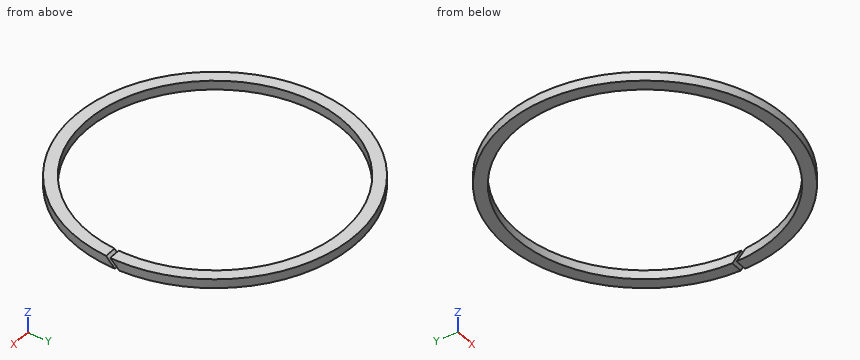
from build123d import *

# Parameters (mm, degrees)
SKETCH1_R               = 46.5
SKETCH1_R_2             = 42.5
BOSS_EXTRUDE1_DEPTH     = 3
CUT_EXTRUDE2_REACH      = 67.829
CUT_EXTRUDE2_END_RADIUS = 46.5


with BuildPart() as part:
    # Sketch1 → Boss-Extrude1 (new body)
    with BuildSketch(Plane.XY):
        Circle(SKETCH1_R)
        Circle(SKETCH1_R_2, mode=Mode.SUBTRACT)
    extrude(amount=BOSS_EXTRUDE1_DEPTH)

    # Cut-Extrude2: up to this cylinder (the profile starts inside it)
    cut_extrude2_end = Plane(origin=(0, 0, -0.237725), z_dir=(0, 0, -1)) * Cylinder(CUT_EXTRUDE2_END_RADIUS, 229.658, mode=Mode.PRIVATE)
    # Sketch2 → Cut-Extrude2 (cut, up to the surface)
    with BuildSketch(Plane(origin=(0, 0, 0), x_dir=(0, 0, -1), z_dir=(1, 0, 0)), mode=Mode.PRIVATE) as cut_extrude2_sk1:
        Polygon((-14.60888812, -13.901781339), (14.377231128, 15.08433791), (15.08433791, 14.377231128), (-13.901781339, -14.60888812), align=None)
    cut_extrude2_tool1 = extrude(cut_extrude2_sk1.sketch, amount=CUT_EXTRUDE2_REACH, mode=Mode.PRIVATE) & cut_extrude2_end
    add(cut_extrude2_tool1.solids().sort_by_distance((0, 0.237725, -0.237725))[0], mode=Mode.SUBTRACT)


solid = part.part
The listing builds one solid part. Answer for the finished solid, in the listing's coordinates (mm). Give positions to 0.01 mm unless a question says otherwise; leave off trailing zeros. Write each loop counter-clockwise with the first axis right and the second up, starting at its lowest first coordinate (ties: lowest second). Pieces come first, ordered by that corner, then holes.
Item 1: Find the intervals of material crossed by line 1 along Y through (x, z) = (0, 1.1); line 2 along Y through (x, z) = (6, 2.45), in increasing order.
Item 2: Section C-C, the plane z = 2.45 is taken. Write down the section's boundary in (x, y), plus the area to 3 significant figures.
Item 3: Section B-B, the plane y = 23.5 is taken. Write down the section's boundary in (x, z), plus the area to 3 significant figures.
Item 4: Section A-A, the plane x = 0 is taken. Write down the section's boundary in (y, z), plus the area to 3 significant figures.
Completed:
1. line 1: y = -46.5 to -42.5, 42.5 to 46.5
1. line 2: y = -46.11 to -42.07, 42.07 to 46.11
2. outline: (42.38, -3.16) arc R42.5 cw (long way) to (42.46, -1.74) - (46.47, -1.74) arc R46.5 ccw (long way) to (46.39, -3.16) - close
2. area: 1,110 mm2
3. outline: (-40.12, 0) - (-35.41, 0) - (-35.41, 3) - (-40.12, 3) - close; (35.41, 0) - (40.12, 0) - (40.12, 3) - (35.41, 3) - close
3. area: 28.3 mm2
4. outline: (-46.5, 0) - (-42.5, 0) - (-42.5, 3) - (-46.5, 3) - close; (42.5, 0) - (46.5, 0) - (46.5, 3) - (42.5, 3) - close
4. area: 24.0 mm2
